```python
from build123d import *

# Parameters (mm, degrees)
SKETCH1_R           = 7.5
BOSS_EXTRUDE1_DEPTH = 6.68
SKETCH2_R           = 2.45
BOSS_EXTRUDE2_DEPTH = 4
SWEEP1_PITCH        = 4
SKETCH6_R           = 1.5
CUT_EXTRUDE1_DEPTH  = 17.75
FILLET2_R           = 3
FILLET3_R           = 1
FILLET4_R           = 1


with BuildPart() as part:
    # Sketch1 → Boss-Extrude1 (new body)
    with BuildSketch(Plane(origin=(0, 0, 0), x_dir=(1, 0, 0), z_dir=(0, 1, 0))):
        with Locations(Location((0, 0, 0), (0, 0, 270))):
            Circle(SKETCH1_R)
    extrude(amount=BOSS_EXTRUDE1_DEPTH)

    # Sketch2 → Boss-Extrude2 (add)
    with BuildSketch(Plane.XZ):
        with Locations(Location((0, 0, 0), (0, 0, 270))):
            Circle(SKETCH2_R)
    extrude(amount=BOSS_EXTRUDE2_DEPTH)

    # Sweep1: the profile of Sketch4 screwed along a right-hand helix of 1 turns, 12 arcs to a turn; built about Z, then put on its axis
    sweep1_z = Axis((0, 0, 0), (0, 0, 1))
    sweep1_corners = [(2.45, 0, 0), (2.45, 0, -0.75), (3.95, 0, 0), (2.45, 0, 0.75)]
    with BuildLine(mode=Mode.PRIVATE) as sweep1_profile:
        Line(sweep1_corners[0], sweep1_corners[1])
        Line(sweep1_corners[1], sweep1_corners[2])
        Line(sweep1_corners[2], sweep1_corners[3])
        Line(sweep1_corners[3], sweep1_corners[0])
    sweep1_cap = Face(sweep1_profile.wire())
    sweep1_turn_angles = [0, 15, 30, 45, 60, 75, 90, 105, 120, 135, 150, 165, 180, 195, 210, 225, 240, 255, 270, 285, 300, 315, 330, 345, 360]
    sweep1_turn_weights = [1, 0.9659258262890683, 1, 0.9659258262890683, 1, 0.9659258262890683, 1, 0.9659258262890683, 1, 0.9659258262890683, 1, 0.9659258262890683, 1, 0.9659258262890683, 1, 0.9659258262890683, 1, 0.9659258262890683, 1, 0.9659258262890683, 1, 0.9659258262890683, 1, 0.9659258262890683, 1]
    sweep1_turn_rails = [Edge.make_bspline([Vector(p[0], p[1], 0).rotate(sweep1_z, sweep1_turn_angles[k]) / sweep1_turn_weights[k] + Vector(0, 0, p[2] + SWEEP1_PITCH * sweep1_turn_angles[k] / 360) for k in range(25)], [0, 0, 0, 1, 1, 2, 2, 3, 3, 4, 4, 5, 5, 6, 6, 7, 7, 8, 8, 9, 9, 10, 10, 11, 11, 12, 12, 12], 2, sweep1_turn_weights) for p in sweep1_corners]
    sweep1_turn_sides = [Face.make_surface_from_curves(sweep1_turn_rails[p[0]], sweep1_turn_rails[p[1]]) for p in [(0, 1), (1, 2), (2, 3), (3, 0)]]
    sweep1 = Plane(origin=(0, -4, 0), x_dir=(-1, 0, 0), z_dir=(0, 1, 0)) * Solid(Shell([*sweep1_turn_sides, sweep1_cap, sweep1_cap.rotate(sweep1_z, 360).moved(Location((0, 0, SWEEP1_PITCH * 360 / 360)))]))
    add(sweep1)

    # Sketch6 → Cut-Extrude1 (cut)
    with BuildSketch(Plane(origin=(0, 6.68, 0), x_dir=(1, 0, 0), z_dir=(0, 1, 0))):
        with Locations((0, 7.5)):
            Circle(SKETCH6_R)
        with Locations((7.132923872, 2.317627458)):
            Circle(SKETCH6_R)
        with Locations((4.408389392, -6.067627458)):
            Circle(SKETCH6_R)
        with Locations((-4.408389392, -6.067627458)):
            Circle(SKETCH6_R)
        with Locations((-7.132923872, 2.317627458)):
            Circle(SKETCH6_R)
    extrude(amount=-CUT_EXTRUDE1_DEPTH, mode=Mode.SUBTRACT)

    # Fillet2
    fillet2_edges = [part.edges().sort_by_distance(p)[0] for p in [
        (1.492481156, 3.34, -7.35),
        (-1.492481156, 3.34, -7.35),
        (7.451467436, 3.34, -0.85184098),
        (6.529063354, 3.34, -3.690708837),
        (3.112778986, 3.34, 6.823533321),
        (5.527664223, 3.34, 5.069016496),
        (-5.527664223, 3.34, 5.069016496),
        (-3.112778986, 3.34, 6.823533321),
        (-6.529063354, 3.34, -3.690708837),
        (-7.451467436, 3.34, -0.85184098),
    ]]
    fillet(fillet2_edges, radius=FILLET2_R)

    # Fillet3
    fillet3_edges = [part.edges().sort_by_distance(p)[0] for p in [
        (-7.132923872, 6.68, 2.317627458),
        (0, 6.68, -6),
        (-4.408389392, 6.68, -6.067627458),
        (-5.706339098, 6.68, -1.854101966),
        (-3.526711514, 6.68, 4.854101966),
        (0, 6.68, 7.5),
        (3.526711514, 6.68, 4.854101966),
        (7.132923872, 6.68, 2.317627458),
        (5.706339098, 6.68, -1.854101966),
        (4.408389392, 6.68, -6.067627458),
        (-7.188301553, 6.68, 0.279858502),
        (-5.650961417, 6.68, -4.451587926),
        (-2.487468593, 6.68, -6.75),
        (2.487468593, 6.68, -6.75),
        (5.650961417, 6.68, -4.451587926),
        (7.188301553, 6.68, 0.279858502),
        (5.979954817, 6.68, 3.998767358),
        (1.955146088, 6.68, 6.922962066),
        (-1.955146088, 6.68, 6.922962066),
        (-5.979954817, 6.68, 3.998767358),
    ]]
    fillet(fillet3_edges, radius=FILLET3_R)

    # Fillet4
    fillet4_edges = [part.edges().sort_by_distance(p)[0] for p in [
        (-7.132923872, 0, 2.317627458),
        (-3.526711514, 0, 4.854101966),
        (-4.408389392, 0, -6.067627458),
        (0, 0, -6),
        (4.408389392, 0, -6.067627458),
        (5.706339098, 0, -1.854101966),
        (7.132923872, 0, 2.317627458),
        (3.526711514, 0, 4.854101966),
        (0, 0, 7.5),
        (-5.706339098, 0, -1.854101966),
        (-7.188301553, 0, 0.279858502),
        (-5.650961417, 0, -4.451587926),
        (-2.487468593, 0, -6.75),
        (2.487468593, 0, -6.75),
        (5.650961417, 0, -4.451587926),
        (7.188301553, 0, 0.279858502),
        (5.979954817, 0, 3.998767358),
        (1.955146088, 0, 6.922962066),
        (-1.955146088, 0, 6.922962066),
        (-5.979954817, 0, 3.998767358),
    ]]
    fillet(fillet4_edges, radius=FILLET4_R)


solid = part.part
```
Input: part model. Units: mm. Frame: model coordinates. A direction names the side the tool comes from. Give positions to 0.01 mm unless a question says otherwise; leave off trailing zeros. Return JSON: item names as keys, results as strings.
Item 1: Ray query, probe 1 along Y at (x, z) = (-4.25, -4); probe 2 along Y at (x, z) = (1.75, -2.25); probe 3 along Y at (x, z) = (1.5, -2.25). Return the intervals inside material, ascending.
Solutions:
{"probe 1": "0 to 6.68", "probe 2": "-1.97 to -0.87, 0 to 6.68", "probe 3": "-2 to -0.75, 0 to 6.68"}
Item 2: Access query for faces 4 (the cylindrical face through (0, 3, -6)), 5 (the flat face through (-2.7, 0, 0.3)), 6 (the flat face through (-3, -4, 0)). Directions: +Z, -Z, +X, -X, +Y, -Y. A direction counts if a zero-diameter tool reaches every point of the face in a straight line with its end or side. Return the directions, or none.
Solutions:
{"face 4": "-Z, +Y, -Y", "face 5": "none", "face 6": "-Z, -X, -Y"}
Item 3: Pull-direction query (Z, two-part tool) for faces 1 (the cylindrical face through (3.537, 3.373, 4.847)), 2 (the cylindrical face through (5.7, 3.37, -1.87)), 3 (the flat face through (0, -4, 0)); classes: +Z half, -Z half, draft (parallel to the pull), parting line (faces both ways), or undercut.
Solutions:
{"face 1": "+Z half", "face 2": "undercut", "face 3": "draft"}
Item 4: First-contact query: P1, Ø3, axis at y = 2, z = -1.5, coming from the +X side; P2, Ø2.5, axis at x = -0.5, z = 1, coming from the -Y side; P3, Ø5, axis at x = 3, y = -2, coming from the -Z side. Flat tips, straight axial feed; report the tip coordinate or a pass-through.
Solutions:
{"P1": "x = 7.08", "P2": "y = -4", "P3": "z = -6.6"}
